```python
from build123d import *

# Parameters (mm, degrees)
SKETCH2_W          = 5
SKETCH2_H          = 100
CUT_EXTRUDE1_DEPTH = 154.717289203
FILLET1_R          = 6
CHAMFER1_SIZE      = 5
CHAMFER2_SIZE      = 2.5
FILLET4_R          = 2
CIRPATTERN1_START  = 72.698022634
CIRPATTERN1_DEPTH  = 9.851977366
SKETCH4_R          = 15
CUT_EXTRUDE2_DEPTH = 100


# Read off the part's stored shape, not the designer's step: CirPattern1
with BuildPart() as part:
    # Sketch2 → Revolve1 (revolve)
    with BuildSketch(Plane(origin=(0, 0, 0), x_dir=(0, 0, -1), z_dir=(1, 0, 0)), mode=Mode.PRIVATE) as revolve1_sk:
        with Locations((-80.05, 50)):
            Rectangle(SKETCH2_W, SKETCH2_H)
    revolve(revolve1_sk.sketch.rotate(Axis((0, -5, 0), (0, 1, 0)), 180), axis=Axis((0, -5, 0), (0, 1, 0)))

    # Sketch3 → Cut-Extrude1 (cut, through all)
    with BuildSketch(Plane(origin=(0, 0, 0), x_dir=(0, 0, -1), z_dir=(1, 0, 0))):
        with BuildLine():
            Line((-6, 100), (6, 100))
            Line((6, 100), (6, 20))
            Line((6, 20), (-21, 20))
            ThreePointArc((-21, 20), (-27, 26), (-21, 32))
            Line((-21, 32), (-6, 32))
            Line((-6, 32), (-6, 100))
        make_face()
    extrude(amount=-CUT_EXTRUDE1_DEPTH, mode=Mode.SUBTRACT)

    # Fillet1
    fillet1_edges = [part.edges().sort_by_distance(p)[0] for p in [
        (-79.824602438, 20, -6),
    ]]
    fillet(fillet1_edges, radius=FILLET1_R)

    # Chamfer1
    chamfer1_edges = [part.edges().sort_by_distance(p)[0] for p in [
        (-79.824602438, 100, -6),
        (-79.824602438, 100, 6),
    ]]
    chamfer(chamfer1_edges, length=CHAMFER1_SIZE)

    # Chamfer2
    chamfer2_edges = [part.edges().sort_by_distance(p)[0] for p in [
        (58.596298945, 100, 50.798388262),
    ]]
    chamfer(chamfer2_edges, length=CHAMFER2_SIZE)

    # Fillet4
    fillet4_edges = [part.edges().sort_by_distance(p)[0] for p in [
        (-79.824602438, 32, 6),
    ]]
    fillet(fillet4_edges, radius=FILLET4_R)

    # CirPattern1 outline → CirPattern1 (cut)
    with BuildSketch(Plane.YZ.offset(CIRPATTERN1_START)):
        with BuildLine():
            ThreePointArc((26, 6), (21.757359313, 4.242640687), (20, 0))
            Line((20, 0), (20, -21))
            ThreePointArc((20, -21), (26, -27), (32, -21))
            Line((32, -21), (32, -8))
            ThreePointArc((32, -8), (32.585786438, -6.585786438), (34, -6))
            Line((34, -6), (95, -6))
            Line((95, -6), (100, -11))
            Line((100, -11), (100, 11))
            Line((100, 11), (95, 6))
            Line((95, 6), (26, 6))
        make_face()
    extrude(amount=CIRPATTERN1_DEPTH, mode=Mode.SUBTRACT)

    # Sketch4 → Cut-Extrude2 (cut)
    with BuildSketch(Plane.XY):
        with Locations(Location((0, 50, 0), (0, 0, 90))):
            Circle(SKETCH4_R)
    extrude(amount=-CUT_EXTRUDE2_DEPTH, mode=Mode.SUBTRACT)


solid = part.part
```
The listing builds one solid part. Answer for the finished solid, in the listing's coordinates (mm). A direction names the side the tool comes from. Round coordinates to 2 decimals unless told otherwise and drop trailing zeros. Write each loop counter-clockwise with the first axis right and the second up, starting at its lowest first coordinate (ties: lowest second). Pieces come first, ordered by that corner, then holes. Notation, with made-up numbers: (27, 26) -> (33, 26) arc R19 cw to (33, 33) -> close; hole circle Ø6 at (56, -40). An arc over 180 degrees is marked (long way). Answer as a JSON object with one key per item and string values. Group by question number.
Q1. Which of the six approach directions +Z, -Z, +X, -X, +Y, -Y give full straight-line access (tool end or side, diameter ignored) to faces 1 (the face through (79, 20, -10)), 2 (the face through (-76, 26, 27)), 3 (the face through (80, 64, -6))?
Q2. Straight lines are drawn through the part: line 1 along X through (y, z) = (29, -52.5); line 2 along Z through (x, y) = (-4, 20); line 3 along X through (y, z) = (65, 18.5). For each, find the intervals that lie inside material, in ascending order.
Q3. Each of these flat-tipped pins is pushed along its axis until it touches: pin 1 Ø4 at (x, z) = (-77.5, 15) entering from -Y; pin 2 Ø10 at (y, z) = (84.5, -18.5) entering from +X; pin 3 Ø6 at (y, z) = (71, -12.5) entering from +X; pin 4 Ø1 at (x, y) = (46, 59.5) entering from +Z. Where does it stop, or does it pass through?
Q4. Section A-A (x = 0) is taken. Write down the section's boundary in (y, z).
Q5. Section D-D (y = 9) is taken. Write down the section's boundary in (x, z).
Q6. Determine the mould class of faces 4 (the face through (1.589, 97.621, -77.655)), 5 (the face through (-74, 0, -24)), 6 (the face through (80.587, 50.7, 17.895)) for opening direction X: pulls with the +X half, pulls with the -X half, needs draft (parallel to the pull), parting line crosses it, or undercut.
Q7. Section C-C (y = 50) is taken. Write down the section's boundary in (x, z).
Q8. Section B-B (y = 79) is taken. Write down the section's boundary in (x, z), plus the area to 3 significant figures.
Check values:
{
 "1": {"face 1": "+X", "face 2": "-X", "face 3": "+X, -X, +Y"},
 "2": {"line 1": "-63.7 to -57.08, 57.08 to 63.7", "line 2": "-82.45 to -77.45, 77.45 to 82.45", "line 3": "-80.45 to -75.31, 75.31 to 80.45"},
 "3": {"pin 1": "y = 0", "pin 2": "x = 81.44", "pin 3": "x = 82", "pin 4": "z = 68.88"},
 "4": {"outline": "(0, -82.55) -> (35, -82.55) -> (35, -77.55) -> (0, -77.55) -> close; (0, 77.55) -> (97.5, 77.55) -> (100, 80.05) -> (100, 82.55) -> (0, 82.55) -> close; (65, -82.55) -> (100, -82.55) -> (100, -80.05) -> (97.5, -77.55) -> (65, -77.55) -> close"},
 "5": {"outline": "circle Ø165.1 at (0, 0); hole circle Ø155.1 at (0, 0)"},
 "6": {"face 4": "undercut", "face 5": "needs draft", "face 6": "parting line crosses it"},
 "7": {"outline": "(-82.33, -6) arc R82.55 ccw to (-15, -81.18) -> (-15, -76.09) arc R77.55 cw to (-77.32, -6) -> close; (-82.33, 6) -> (-77.32, 6) arc R77.55 cw to (77.32, 6) -> (82.33, 6) arc R82.55 ccw to start; (15, -81.18) arc R82.55 ccw to (82.33, -6) -> (77.32, -6) arc R77.55 cw to (15, -76.09) -> close"},
 "8": {"outline": "(-82.33, -6) arc R82.55 ccw to (82.33, -6) -> (77.32, -6) arc R77.55 cw to (-77.32, -6) -> close; (-82.33, 6) -> (-77.32, 6) arc R77.55 cw to (77.32, 6) -> (82.33, 6) arc R82.55 ccw to start", "area": "2,390 mm^2"}
}
